Geometry check sheet. Reference: the model listing, model coordinates, mm. Round coordinates to 2 decimals unless told otherwise and drop trailing zeros. Loops run counter-clockwise (first coordinate to the right, second up) from the corner with the lowest first, then second, coordinate; pieces in that order, holes last. Notation, with made-up numbers: (-15.75, -39) - (24.25, -39) arc R17 cw to (24.25, -31) - close; hole circle Ø11 at (38, 63.5). An arc over 180 degrees is marked (long way). Write item = value, one per line.
```python
from build123d import *

# Parameters (mm, degrees)
F0_R     = 62.5
F0_R_2   = 0.95
F1_DEPTH = 3


with BuildPart() as f1:
    # F0 (on Top) → F1 (new body)
    with BuildSketch(Plane.XY):
        with Locations((-11.4963501692, 27.9728826135)):
            Circle(F0_R)
        with Locations((-54.0467362732, -14.4027499996)):
            Circle(F0_R_2, mode=Mode.SUBTRACT)
        with Locations((-27.1582491696, -30.0006847829)):
            Circle(F0_R_2, mode=Mode.SUBTRACT)
        with Locations((-69.5338817827, 12.5497013212)):
            Circle(F0_R_2, mode=Mode.SUBTRACT)
        with Locations((3.9268311232, -30.064649)):
            Circle(F0_R_2, mode=Mode.SUBTRACT)
        with Locations((30.8792824439, -14.5775034905)):
            Circle(F0_R_2, mode=Mode.SUBTRACT)
        with Locations((46.4772172272, 12.3109836131)):
            Circle(F0_R_2, mode=Mode.SUBTRACT)
        with Locations((-69.4699175656, 43.6347816139)):
            Circle(F0_R_2, mode=Mode.SUBTRACT)
        with Locations((-53.8719827823, 70.5232687176)):
            Circle(F0_R_2, mode=Mode.SUBTRACT)
        with Locations((-26.9195314615, 86.010414227)):
            Circle(F0_R_2, mode=Mode.SUBTRACT)
        with BuildLine():
            ThreePointArc((35.0970928529, 61.6671116053), (37.5498519583, 57.9848811619), (39.7122301293, 54.1249629097))
            ThreePointArc((39.7122301293, 54.1249629097), (44.4086736085, 41.4219835656), (46.0036498308, 27.9728826135))
            ThreePointArc((46.0036498308, 27.9728826135), (39.707498158, 1.8115386785), (22.1978788226, -18.6205604085))
            ThreePointArc((22.1978788226, -18.6205604085), (18.5156483792, -21.073319514), (14.655730127, -23.2356976849))
            ThreePointArc((14.655730127, -23.2356976849), (-24.9555645945, -27.9297071928), (-58.0897931912, -5.7213463782))
            ThreePointArc((-58.0897931912, -5.7213463782), (-60.5425522967, -2.0391159348), (-62.7049304676, 1.8208023173))
            ThreePointArc((-62.7049304676, 1.8208023173), (-67.3989399755, 41.4320970388), (-45.190579161, 74.5663256356))
            ThreePointArc((-45.190579161, 74.5663256356), (-41.5083487176, 77.019084741), (-37.6484304654, 79.181462912))
            ThreePointArc((-37.6484304654, 79.181462912), (1.9628642561, 83.8754724199), (35.0970928529, 61.6671116053))
        make_face(mode=Mode.SUBTRACT)
        with Locations((46.5411814443, 43.3960639059)):
            Circle(F0_R_2, mode=Mode.SUBTRACT)
        with Locations((4.1655488312, 85.9464500099)):
            Circle(F0_R_2, mode=Mode.SUBTRACT)
        with Locations((31.0540359349, 70.3485152266)):
            Circle(F0_R_2, mode=Mode.SUBTRACT)
        with BuildLine():
            ThreePointArc((-23.0942292571, 50.6827747459), (-5.5274811632, 52.764465919), (9.1668289102, 42.9155406882))
            Line((9.1668289102, 42.9155406882), (13.2184326512, 45.845473644))
            ThreePointArc((13.2184326512, 45.845473644), (-4.3571146914, 57.6255606847), (-25.3683231959, 55.1356947718))
            Line((-25.3683231959, 55.1356947718), (-23.0942292571, 50.6827747459))
        make_face()
        with BuildLine():
            ThreePointArc((-34.2062423015, 16.3750035257), (-36.2879334746, 33.9417516195), (-26.4390082438, 48.6360616929))
            Line((-26.4390082438, 48.6360616929), (-29.3689411996, 52.6876654339))
            ThreePointArc((-29.3689411996, 52.6876654339), (-41.1490282404, 35.1121180913), (-38.6591623275, 14.1009095869))
            Line((-38.6591623275, 14.1009095869), (-34.2062423015, 16.3750035257))
        make_face()
        with BuildLine():
            Line((2.3756228575, 0.8100704552), (0.1015289187, 5.2629904812))
            ThreePointArc((0.1015289187, 5.2629904812), (-17.4652191752, 3.1812993081), (-32.1595292485, 13.0302245389))
            Line((-32.1595292485, 13.0302245389), (-36.2111329896, 10.1002915831))
            ThreePointArc((-36.2111329896, 10.1002915831), (-18.6355856469, -1.6797954576), (2.3756228575, 0.8100704552))
        make_face()
        with BuildLine():
            ThreePointArc((11.2135419632, 39.5707617014), (13.2963125496, 33.937266514), (14.0036498308, 27.9728826135))
            ThreePointArc((14.0036498308, 27.9728826135), (11.2114434368, 16.3708953032), (3.4463079054, 7.3097035342))
            Line((3.4463079054, 7.3097035342), (6.3762408612, 3.2580997931))
            ThreePointArc((6.3762408612, 3.2580997931), (15.663951987, 14.0959958306), (19.0036498308, 27.9728826135))
            ThreePointArc((19.0036498308, 27.9728826135), (18.1576189651, 35.1067535534), (15.6664619891, 41.8448556402))
            Line((15.6664619891, 41.8448556402), (11.2135419632, 39.5707617014))
        make_face()
        with BuildLine():
            ThreePointArc((13.2184326512, 45.845473644), (14.5194613941, 43.8922905392), (15.6664619891, 41.8448556402))
            Line((15.6664619891, 41.8448556402), (21.0287945872, 44.5833840638))
            ThreePointArc((21.0287945872, 44.5833840638), (19.6553594594, 47.0350122708), (18.097488796, 49.3737820141))
            Line((18.097488796, 49.3737820141), (13.2184326512, 45.845473644))
        make_face()
        with BuildLine():
            ThreePointArc((-29.3689411996, 52.6876654339), (-27.4157580948, 53.9886941768), (-25.3683231959, 55.1356947718))
            Line((-25.3683231959, 55.1356947718), (-28.1068516195, 60.4980273699))
            ThreePointArc((-28.1068516195, 60.4980273699), (-30.5584798265, 59.1245922421), (-32.8972495697, 57.5667215788))
            Line((-32.8972495697, 57.5667215788), (-29.3689411996, 52.6876654339))
        make_face()
        with BuildLine():
            Line((9.9045492314, -1.6209563517), (6.3762408612, 3.2580997931))
            ThreePointArc((6.3762408612, 3.2580997931), (4.4230577565, 1.9570710503), (2.3756228575, 0.8100704552))
            Line((2.3756228575, 0.8100704552), (5.1141512811, -4.5522621428))
            ThreePointArc((5.1141512811, -4.5522621428), (7.5657794881, -3.178827015), (9.9045492314, -1.6209563517))
        make_face()
        with BuildLine():
            Line((-41.0901891344, 6.571983213), (-36.2111329896, 10.1002915831))
            ThreePointArc((-36.2111329896, 10.1002915831), (-37.5121617325, 12.0534746879), (-38.6591623275, 14.1009095869))
            Line((-38.6591623275, 14.1009095869), (-44.0214949255, 11.3623811633))
            ThreePointArc((-44.0214949255, 11.3623811633), (-42.6480597977, 8.9107529563), (-41.0901891344, 6.571983213))
        make_face()
        with BuildLine():
            Line((21.0287945872, 44.5833840638), (15.6664619891, 41.8448556402))
            ThreePointArc((15.6664619891, 41.8448556402), (18.1576189651, 35.1067535534), (19.0036498308, 27.9728826135))
            ThreePointArc((19.0036498308, 27.9728826135), (15.663951987, 14.0959958306), (6.3762408612, 3.2580997931))
            Line((6.3762408612, 3.2580997931), (9.9045492314, -1.6209563517))
            ThreePointArc((9.9045492314, -1.6209563517), (21.0257890743, 11.3564973604), (25.024791651, 27.9728826135))
            ThreePointArc((25.024791651, 27.9728826135), (24.0117420368, 36.5150830175), (21.0287945872, 44.5833840638))
        make_face()
        with BuildLine():
            Line((5.1141512811, -4.5522621428), (2.3756228575, 0.8100704552))
            ThreePointArc((2.3756228575, 0.8100704552), (-18.6355856469, -1.6797954576), (-36.2111329896, 10.1002915831))
            Line((-36.2111329896, 10.1002915831), (-41.0901891344, 6.571983213))
            ThreePointArc((-41.0901891344, 6.571983213), (-20.0449741486, -7.5336636549), (5.1141512811, -4.5522621428))
        make_face()
        with BuildLine():
            ThreePointArc((-38.6591623275, 14.1009095869), (-41.1490282404, 35.1121180913), (-29.3689411996, 52.6876654339))
            Line((-29.3689411996, 52.6876654339), (-32.8972495697, 57.5667215788))
            ThreePointArc((-32.8972495697, 57.5667215788), (-47.0028964376, 36.5215065929), (-44.0214949255, 11.3623811633))
            Line((-44.0214949255, 11.3623811633), (-38.6591623275, 14.1009095869))
        make_face()
        with BuildLine():
            ThreePointArc((-25.3683231959, 55.1356947718), (-4.3571146914, 57.6255606847), (13.2184326512, 45.845473644))
            Line((13.2184326512, 45.845473644), (18.097488796, 49.3737820141))
            ThreePointArc((18.097488796, 49.3737820141), (-2.9477261898, 63.479428882), (-28.1068516195, 60.4980273699))
            Line((-28.1068516195, 60.4980273699), (-25.3683231959, 55.1356947718))
        make_face()
        with BuildLine():
            Line((-58.0897931912, -5.7213463782), (-41.0901891344, 6.571983213))
            ThreePointArc((-41.0901891344, 6.571983213), (-42.6480597977, 8.9107529563), (-44.0214949255, 11.3623811633))
            Line((-44.0214949255, 11.3623811633), (-62.7049304676, 1.8208023173))
            ThreePointArc((-62.7049304676, 1.8208023173), (-60.5425522967, -2.0391159348), (-58.0897931912, -5.7213463782))
        make_face()
        with BuildLine():
            Line((22.1978788226, -18.6205604085), (9.9045492314, -1.6209563517))
            ThreePointArc((9.9045492314, -1.6209563517), (7.5657794881, -3.178827015), (5.1141512811, -4.5522621428))
            Line((5.1141512811, -4.5522621428), (14.655730127, -23.2356976849))
            ThreePointArc((14.655730127, -23.2356976849), (18.5156483792, -21.073319514), (22.1978788226, -18.6205604085))
        make_face()
        with BuildLine():
            ThreePointArc((18.097488796, 49.3737820141), (19.6553594594, 47.0350122708), (21.0287945872, 44.5833840638))
            Line((21.0287945872, 44.5833840638), (39.7122301293, 54.1249629097))
            ThreePointArc((39.7122301293, 54.1249629097), (37.5498519583, 57.9848811619), (35.0970928529, 61.6671116053))
            Line((35.0970928529, 61.6671116053), (18.097488796, 49.3737820141))
        make_face()
        with BuildLine():
            ThreePointArc((-32.8972495697, 57.5667215788), (-30.5584798265, 59.1245922421), (-28.1068516195, 60.4980273699))
            Line((-28.1068516195, 60.4980273699), (-37.6484304654, 79.181462912))
            ThreePointArc((-37.6484304654, 79.181462912), (-41.5083487176, 77.019084741), (-45.190579161, 74.5663256356))
            Line((-45.190579161, 74.5663256356), (-32.8972495697, 57.5667215788))
        make_face()
    extrude(amount=F1_DEPTH)


solid = f1.part
```
(1) Scan lines: L1, parallel to Y at x = -8, z = 1.5; L2, parallel to X at y = 38, z = 1.6; L3, parallel to X at y = 67, z = 2.35. Record each from-to range of solid material in increasing order. Write a range as [from, to].
Answers follow:
L1 = [-34.43, -29.42], [-8.38, 2.71], [53.23, 64.33], [85.37, 90.38]
L2 = [-73.19, -68.12], [-46.61, -34.94], [11.95, 23.62], [45.12, 50.19]
L3 = [-60.31, -53.72], [-39.72, -31.43], [30.73, 37.32]
(2) Section check B-B (x = 43). Enter the section's corners in (y, z), then the cut area to 3 significant figures.
Answers follow:
outline = (-2.63, 0) - (9.63, 0) - (9.63, 3) - (-2.63, 3) - close; (46.31, 0) - (58.57, 0) - (58.57, 3) - (46.31, 3) - close
area = 73.6 mm²
(3) Section check C-C (z = 2.05). State how many separate pieces and enclosed holes the cut face has, then the cut area to 3 significant figures.
Answers follow:
separate_pieces = 1
enclosed_holes = 17
area = 4,520 mm²
(4) Gauge pin test, flat ends, axial feed: pin 1 (1.7 mm diameter, centred on x = -69.47, y = 43.63, fed in from +Z); pin 2 (1.5 mm diameter, centred on y = -7, z = 2.5, fed in from +X). Record the tip position at first contact, or that the pin passes through.
Answers follow:
pin_1 = through
pin_2 = 40.8
(5) Mould release check, pull along X, two halves, no side actions. Record for faces 1 (the cylindrical face through (-19.63, 89.94, 1.48)), 2 (the flat face through (26.72, 55.61, 1.48)): pulls with the +X half, pulls with the -X half, needs draft (parallel to the pull), parting line crosses it, or undercut.
Answers follow:
face_1 = parting line crosses it
face_2 = undercut
(6) Section check A-A (y = 35). Enter the section's corners in (x, z).
Answers follow:
outline = (-73.6, 0) - (-68.57, 0) - (-68.57, 3) - (-73.6, 3) - close; (-47.34, 0) - (-36.01, 0) - (-36.01, 3) - (-47.34, 3) - close; (13.02, 0) - (24.34, 0) - (24.34, 3) - (13.02, 3) - close; (45.57, 0) - (50.61, 0) - (50.61, 3) - (45.57, 3) - close
